Geometry check sheet. Reference: the model listing, model coordinates, mm. A direction names the side the tool comes from. Round coordinates to 2 decimals unless told otherwise and drop trailing zeros. Order: outer loops, then holes, each group sorted by start corner. A loop starts at its lowest first (then second) coordinate and runs counter-clockwise, first axis right, second up.
```python
from build123d import *

# Parameters (mm, degrees)
BOSS_EXTRUDE1_DEPTH = 6.5
SKETCH2_W           = 60.158889846
SKETCH2_H           = 120
BOSS_EXTRUDE3_DEPTH = 5
SKETCH6_R           = 3
CUT_EXTRUDE7_DEPTH  = 5.1
BOSS_EXTRUDE4_DEPTH = 31
CUT_EXTRUDE8_REACH  = 119.187
SKETCH11_W          = 5.5
SKETCH11_H          = 10.5
CUT_EXTRUDE11_REACH = 119.187
SKETCH14_R          = 3
SKETCH29_R          = 1.5
BOSS_EXTRUDE6_DEPTH = 5
RIB6_START          = -2.5
RIB6_DEPTH          = 5
CUT_EXTRUDE14_REACH = 118.769
CUT_EXTRUDE15_REACH = 119.187
SKETCH66_W          = 8
SKETCH66_H          = 13
FILLET3_R           = 4
FILLET4_R           = 0.5


# Read off the part's stored shape, not the designer's step: Rib6
with BuildPart() as part:
    # Sketch1 → Boss-Extrude1 (new body)
    with BuildSketch(Plane.XY):
        with BuildLine():
            Line((-15.5, -30), (-15.5, 30))
            Line((-15.5, 30), (15.5, 30))
            Line((15.5, 30), (15.5, -30))
            Line((15.5, -30), (15.5, -90))
            Line((15.5, -90), (-30, -90))
            add(Edge.make_bspline(
                [(-15.5, -30), (-15.682751911, -39.304401058), (-30, -90)],
                knots=[0.243669215, 0.243669215, 0.243669215, 1, 1, 1], degree=2))
        make_face()
    extrude(amount=BOSS_EXTRUDE1_DEPTH)

    # Sketch2 → Boss-Extrude3 (add)
    with BuildSketch(Plane(origin=(0, -22.5, -38.97114317), x_dir=(1, 0, 0), z_dir=(0, 0.500000000000001, 0.866025403784438))):
        with Locations((0.079444923, -21.192286341)):
            Rectangle(SKETCH2_W, SKETCH2_H)
    extrude(amount=BOSS_EXTRUDE3_DEPTH)

    # Sketch6 → Cut-Extrude7 (cut)
    with BuildSketch(Plane(origin=(0, -22.5, -38.97114317), x_dir=(-1, 0, 0), z_dir=(0, -0.5000000000000012, -0.866025403784438))):
        with Locations(Location((-20.158889846, -30.893082241, 0), (0, 0, 90))):
            Circle(SKETCH6_R)
        with Locations(Location((20, -30.893082241, 0), (0, 0, 90))):
            Circle(SKETCH6_R)
        with Locations(Location((-0.079444923, 28.807713659, 0), (0, 0, 90))):
            Circle(SKETCH6_R)
    extrude(amount=-CUT_EXTRUDE7_DEPTH, mode=Mode.SUBTRACT)

    # Sketch10 → Boss-Extrude4 (add)
    with BuildSketch(Plane(origin=(15.5, 0, 0), x_dir=(0, 0, -1), z_dir=(1, 0, 0))):
        with BuildLine():
            Line((-6.5, 36.5), (-6.5, 30))
            Line((-6.5, 30), (0, 30))
            ThreePointArc((0, 30), (-1.903805922, 34.596194078), (-6.5, 36.5))
        make_face()
    extrude(amount=-BOSS_EXTRUDE4_DEPTH)

    # Sketch11 → Cut-Extrude8 (cut, up to next)
    with BuildSketch(Plane.XY.offset(6.5), mode=Mode.PRIVATE) as cut_extrude8_sk1:
        with Locations((-12.75, 31.25)):
            Rectangle(SKETCH11_W, SKETCH11_H)
    cut_extrude8_tool1 = extrude(cut_extrude8_sk1.sketch, amount=-CUT_EXTRUDE8_REACH, mode=Mode.PRIVATE) & part.part
    add(cut_extrude8_tool1.solids().sort_by_distance((-12.75, 31.25, 6.5))[0], mode=Mode.SUBTRACT)

    # Sketch14 → Cut-Extrude11 (cut, up to next)
    with BuildSketch(Plane.XY.offset(6.5), mode=Mode.PRIVATE) as cut_extrude11_sk1:
        with Locations((-5.5, 16.5)):
            Circle(SKETCH14_R)
    cut_extrude11_tool1 = extrude(cut_extrude11_sk1.sketch, amount=-CUT_EXTRUDE11_REACH, mode=Mode.PRIVATE) & part.part
    # Sketch14 → Cut-Extrude11 (cut, up to next)
    with BuildSketch(Plane.XY.offset(6.5), mode=Mode.PRIVATE) as cut_extrude11_sk2:
        with Locations((-5.5, -5)):
            Circle(SKETCH14_R)
    cut_extrude11_tool2 = extrude(cut_extrude11_sk2.sketch, amount=-CUT_EXTRUDE11_REACH, mode=Mode.PRIVATE) & part.part
    add(cut_extrude11_tool1.solids().sort_by_distance((-5.5, 16.5, 6.5))[0], mode=Mode.SUBTRACT)
    add(cut_extrude11_tool2.solids().sort_by_distance((-5.5, -5, 6.5))[0], mode=Mode.SUBTRACT)

    # Sketch29 → Boss-Extrude6 (add)
    with BuildSketch(Plane(origin=(30.158889846, 0, 0), x_dir=(0, 0, -1), z_dir=(1, 0, 0))):
        with BuildLine():
            Line((-4.298836218, 35.789748924), (54.044872981, 13.608465892))
            Line((54.044872981, 13.608465892), (37.966397208, -14.240271055))
            Line((37.966397208, -14.240271055), (-10.413719231, 25.199050471))
            ThreePointArc((-10.413719231, 25.199050471), (-11.864134131, 33.0971567), (-4.298836218, 35.789748924))
        make_face()
        with Locations(Location((-6.5, 30, 0), (0, 0, 90))):
            Circle(SKETCH29_R, mode=Mode.SUBTRACT)
    extrude(amount=-BOSS_EXTRUDE6_DEPTH)

    # Rib6 outline → Rib6 (add)
    with BuildSketch(Plane(origin=(5, 0, 0), x_dir=(0, 0, -1), z_dir=(1, 0, 0)).offset(RIB6_START)):
        with BuildLine():
            Line((0, -80), (34.010848977, -21.091481564))
            add(Edge.make_bspline(
                [(34.010848977, -21.091481564), (7.27651008, -47.405497337), (0, -7.927359395)],
                knots=[0, 0, 0, 1, 1, 1], degree=2))
            Line((0, -7.927359395), (0, -80))
        make_face()
    extrude(amount=RIB6_DEPTH)

    # Sketch65 → Cut-Extrude14 (cut, up to next)
    with BuildSketch(Plane.ZY.offset(10), mode=Mode.PRIVATE) as cut_extrude14_sk1:
        with BuildLine():
            Line((6.5, 34), (6.5, 26))
            ThreePointArc((6.5, 26), (2.5, 30), (6.5, 34))
        make_face()
    cut_extrude14_tool1 = extrude(cut_extrude14_sk1.sketch, amount=-CUT_EXTRUDE14_REACH, mode=Mode.PRIVATE) & part.part
    add(cut_extrude14_tool1.solids().sort_by_distance((-10, 30, 4.802347))[0], mode=Mode.SUBTRACT)

    # Sketch66 → Cut-Extrude15 (cut, up to next)
    with BuildSketch(Plane.XY.offset(6.5), mode=Mode.PRIVATE) as cut_extrude15_sk1:
        with Locations((11.5, 9.5)):
            Rectangle(SKETCH66_W, SKETCH66_H)
    cut_extrude15_tool1 = extrude(cut_extrude15_sk1.sketch, amount=-CUT_EXTRUDE15_REACH, mode=Mode.PRIVATE) & part.part
    add(cut_extrude15_tool1.solids().sort_by_distance((11.5, 9.5, 6.5))[0], mode=Mode.SUBTRACT)

    # Fillet3
    fillet3_edges = [part.edges().sort_by_distance(p)[0] for p in [
        (15.5, 16, 3.25),
        (15.5, 3, 3.25),
    ]]
    fillet(fillet3_edges, radius=FILLET3_R)

    # Fillet4
    fillet4_edges = [part.edges().sort_by_distance(p)[0] for p in [
        (7.5, 3, 3.25),
        (7.5, 16, 3.25),
    ]]
    fillet(fillet4_edges, radius=FILLET4_R)


solid = part.part
```
(1) Sectioned sample at B-B, the plane y = -5. Record the cut outline in (x, z).
Returned:
outline: (-30, -49.07) - (30.16, -49.07) - (30.16, -26.63) - (25.16, -26.63) - (25.16, -43.3) - (-30, -43.3) - close; (-15.5, 0) - (-8.5, 0) - (-8.5, 6.5) - (-15.5, 6.5) - close; (-2.5, 0) - (15.5, 0) - (15.5, 6.5) - (-2.5, 6.5) - close
(2) Sectioned sample at A-A, the plane x = -5.5. Give the number of separate pieces and of enclosed holes in the cut face, and give its area (3 significant figures).
Returned:
separate pieces: 3
enclosed holes: 0
area: 1,280 mm2
(3) Depth check by flat-ended pin: P1, Ø3, axis at y = 9, z = 2, coming from the -X side; P2, Ø3, axis at y = 8.5, z = 2.5, coming from the +X side; P3, Ø2, axis at x = 6, z = -50.5, coming from the +Y side. Enter the tip coordinate at first touch or a pass-through.
Returned:
P1: stops at x = -15.5
P2: stops at x = 7.5
P3: stops at y = 9.2
(4) Material ranges on line 1 (Y direction, x = 12.5, z = 4.5); line 2 (X direction, y = 22, z = 4.5); line 3 (Y direction, x = -5, z = 3), recorded low to high.
Returned:
line 1: y = -91.15 to 2.87, 16.13 to 26.54, 33.46 to 36.18
line 2: x = -15.5 to 15.5, 25.16 to 30.16
line 3: y = -92.02 to -7.96, -2.04 to 13.54, 19.46 to 28.06, 31.94 to 35.48
(5) Draft check along Y on faces 1 (the flat face through (27.694, 24.854, -24.465)), 2 (the flat face through (2.5, -44, -9)), 3 (the cylindrical face through (14.297, 17.141, 3.204)), 4 (the cylindrical face through (-22.66, -46.82, -22.08)). Enter one of: released by +Y, released by -Y, zero draft, split by the parting line, or undercut.
Returned:
face 1: released by +Y
face 2: zero draft
face 3: undercut
face 4: undercut
(6) Sectioned sample at C-C, the plane y = 9.5. Record the cut outline in (x, z).
Returned:
outline: (-30, -57.45) - (30.16, -57.45) - (30.16, -8.84) - (25.16, -8.84) - (25.16, -51.67) - (-30, -51.67) - close; (-15.5, 0) - (7.5, 0) - (7.5, 6.5) - (-15.5, 6.5) - close
(7) Set-up check for faces 5 (the cylindrical face through (14.359, 1.797, 3.204)), 6 (the cylindrical face through (2.928, 34.545, 1.854)), 7 (the flat face through (7.5, -44, -9)): record each of +Z, -Z, +X, -X, +Y, -Y from which the full face is reachable in a straight line by a thin tool's end or side.
Returned:
face 5: +Z, +X
face 6: -Z, -X, +Y
face 7: +X, +Y
